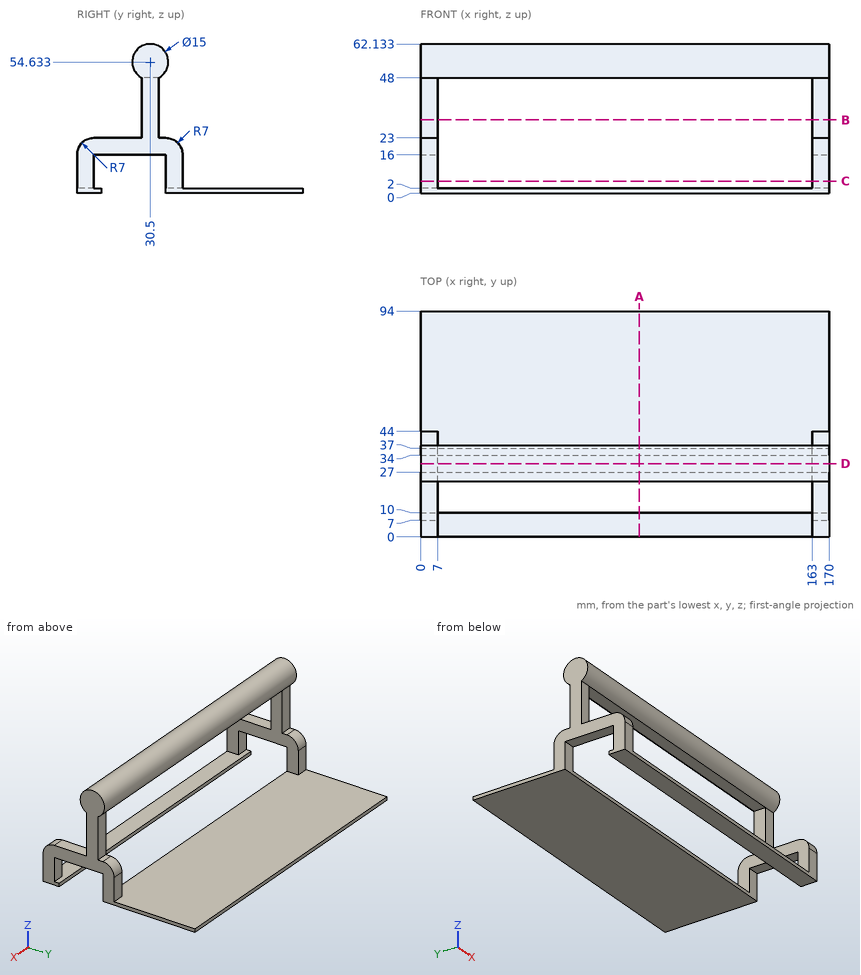
The figure shows three views and two pictorial views of one solid part (mm, origin at its lowest corner). Answer the questions. Coordinates: 2 decimals unless noted, no trailing zeros. Loops run counter-clockwise (first coordinate to the right, second up) from the corner with the lowest first, then second, coordinate; pieces in that order, holes last.
1) Flat-ended cylindrical pins translate along their axes: pin 1 Ø7.5 at (x, y) = (61, 32) entering from -Z; pin 2 Ø8 at (y, z) = (31.5, 43.5) entering from -X; pin 3 Ø3.5 at (x, y) = (3.5, 18) entering from +Z; pin 4 Ø5.5 at (x, z) = (4.5, 37.5) entering from +Y. Find the tip coordinate at first contact, or state that the pin passes through.
2) Find section D-D on y = 30.5. Write down the section's boundary in (x, z), then the cut area to 3 significant figures.
3) Find section C-C on z = 5. Write down the section's boundary in (x, y), then the cut area to 3 significant figures.
4) Find the intervals of material crossed by L1, parallel to X at y = 35, z = 19; L2, parallel to Z at x = 9, y = 77; L3, parallel to Y at x = 40, z = 50, in increasing order.
5) Find section B-B on z = 30.5. Write down the section's boundary in (x, y), then the cut area to 3 significant figures.
6) Find section A-A on x = 91. Write down the section's boundary in (y, z), then the cut area to 3 significant figures.
Values:
1. pin 1: stops at z = 48
1. pin 2: stops at x = 0
1. pin 3: stops at z = 23
1. pin 4: stops at y = 34
2. outline: (0, 16) - (7, 16) - (7, 48) - (163, 48) - (163, 16) - (170, 16) - (170, 62.13) - (0, 62.13) - close
2. area: 2,850 mm2
3. outline: (0, 0) - (7, 0) - (7, 7) - (0, 7) - close; (0, 37) - (7, 37) - (7, 44) - (0, 44) - close; (163, 0) - (170, 0) - (170, 7) - (163, 7) - close; (163, 37) - (170, 37) - (170, 44) - (163, 44) - close
3. area: 196 mm2
4. L1: x = 0 to 7, 163 to 170
4. L2: z = 0 to 2
4. L3: y = 24.6 to 36.4
5. outline: (0, 27) - (7, 27) - (7, 34) - (0, 34) - close; (163, 27) - (170, 27) - (170, 34) - (163, 34) - close
5. area: 98.0 mm2
6. outline: (0, 0) - (10, 0) - (10, 2) - (0, 2) - close; (27, 48) - (34, 48) arc R7.5 ccw (long way) to start; (37, 0) - (94, 0) - (94, 2) - (37, 2) - close
6. area: 307 mm2
